Can you work these out from the model? Positions are in its coordinate system, mm. Face numbers are marked on the shaded views. Give positions to 0.01 mm unless a question says otherwise; leave off trailing zeros. Order: outer loops, then holes, each group sorted by start corner. A loop starts at its lowest first (then second) coordinate and runs counter-clockwise, first axis right, second up. Notation, with made-up numbers: (53.25, -6) -> (78.25, -6) arc R31 cw to (78.25, 32) -> close; hole circle Ø8 at (58.5, -19.5). An arc over 180 degrees is marked (long way). Answer as a JSON object with one key per item and string values.
Autodesk Inventor part; units mm, degrees
ref_plane "YZ Plane" through (0, 0, 0) normal (1, 0, 0) x (0, 1, 0)
ref_plane "XZ Plane" through (0, 0, 0) normal (0, 1, 0) x (-1, 0, 0)
ref_plane "XY Plane" through (0, 0, 0) normal (0, 0, 1) x (1, 0, 0)
sketch "스케치1" plane through (0, 0, 0) normal (1, 0, 0) x (0, 1, 0)
  line L0 (0, 0) -> (0, 20)
  line L1 (0, 20) -> (0, 50)
  line L2 (0, 0) -> (37.3205, 0)
  line L3 (0, 20) -> (17.3205, 20)
  line L4 (0, 50) -> (17.3205, 20)
  line L5 (0, 50) -> (34.641, 50) construction
  line L6 (17.3205, 20) -> (37.3205, 0)
  line L7 (17.3205, 20) -> (45.6048, 20) construction
  dimension "d0" = 20
  dimension "d1" = 30
  dimension "d2" = 60
  dimension "d3" = 45
extrude "돌출1" add sketch "스케치1" along normal blind 8
sketch "스케치2" plane through (8, 0, 0) normal (1, 0, 0) x (0, 0, -1)
  line L0 (-20, 17.3205) -> (-50, 0)
  line L1 (-50, 0) -> (0, 0)
  line L2 (0, 0) -> (0, 37.3205)
  line L3 (0, 37.3205) -> (-20, 17.3205)
  line L4 (-35.0718, 4) -> (-17.5439, 14.1197)
  line L5 (-17.5439, 14.1197) -> (-4, 27.6637)
  line L6 (-4, 27.6637) -> (-4, 4)
  line L7 (-4, 4) -> (-35.0718, 4)
  dimension "d6" = 4
extrude "돌출2" cut sketch "스케치2" against normal blind 8 contours L4 L5 L6 L7
sketch "스케치5" plane through (0, 0, 0) normal (0, -1, 0) x (1, 0, 0)
  arc A0 (157.7, 33) -> (156.7, 34) centre (156.7, 33) ccw
  line L0 (157.7, 33) -> (157.7, 24)
  arc A1 (156.7, 23) -> (157.7, 24) centre (156.7, 24) ccw
  line L1 (156.7, 23) -> (136.7, 23)
  arc A2 (135.7, 24) -> (136.7, 23) centre (136.7, 24) ccw
  line L2 (135.7, 24) -> (135.7, 33)
  arc A3 (136.7, 34) -> (135.7, 33) centre (136.7, 33) ccw
  line L3 (136.7, 34) -> (156.7, 34)
  arc A4 (-61.9, 33) -> (-62.9, 34) centre (-62.9, 33) ccw
  line L4 (-61.9, 33) -> (-61.9, 24)
  arc A5 (-62.9, 23) -> (-61.9, 24) centre (-62.9, 24) ccw
  line L5 (-62.9, 23) -> (-82.9, 23)
  arc A6 (-83.9, 24) -> (-82.9, 23) centre (-82.9, 24) ccw
  line L6 (-83.9, 24) -> (-83.9, 33)
  arc A7 (-82.9, 34) -> (-83.9, 33) centre (-82.9, 33) ccw
  line L7 (-82.9, 34) -> (-62.9, 34)
  arc A8 (-61.9, -244) -> (-62.9, -243) centre (-62.9, -244) ccw
  line L8 (-61.9, -244) -> (-61.9, -253)
  arc A9 (-62.9, -254) -> (-61.9, -253) centre (-62.9, -253) ccw
  line L9 (-62.9, -254) -> (-82.9, -254)
  arc A10 (-83.9, -253) -> (-82.9, -254) centre (-82.9, -253) ccw
  line L10 (-83.9, -253) -> (-83.9, -244)
  arc A11 (-82.9, -243) -> (-83.9, -244) centre (-82.9, -244) ccw
  line L11 (-82.9, -243) -> (-62.9, -243)
  arc A12 (136.7, -243) -> (135.7, -244) centre (136.7, -244) ccw
  line L12 (136.7, -243) -> (156.7, -243)
  arc A13 (157.7, -244) -> (156.7, -243) centre (156.7, -244) ccw
  line L13 (157.7, -244) -> (157.7, -253)
  arc A14 (156.7, -254) -> (157.7, -253) centre (156.7, -253) ccw
  line L14 (156.7, -254) -> (136.7, -254)
  arc A15 (135.7, -253) -> (136.7, -254) centre (136.7, -253) ccw
  line L15 (135.7, -253) -> (135.7, -244)
  line L16 (-98.1, 40) -> (171.9, 40)
  line L17 (-98.1, 0) -> (-98.1, 40)
  line L18 (-58.1, 0) -> (-98.1, 0)
  line L19 (-58.1, -220) -> (-58.1, 0)
  line L20 (-98.1, -220) -> (-58.1, -220)
  line L21 (-98.1, -260) -> (-98.1, -220)
  line L22 (171.9, -260) -> (-98.1, -260)
  line L23 (171.9, -220) -> (171.9, -260)
  line L24 (131.9, -220) -> (171.9, -220)
  line L25 (131.9, 0) -> (131.9, -220)
  line L26 (171.9, 0) -> (131.9, 0)
  line L27 (171.9, 40) -> (171.9, 0)
  circle A16 centre (4, 14.0286) radius 1.25
  circle A17 centre (4, 36.0286) radius 1.25
  point P0 (0, 0)
  dimension "d17" = 2.5
  dimension "d18" = 2.5
extrude "돌출5" cut sketch "스케치5" against normal blind 4.1 contours A16 | A17
sketch "스케치8" plane through (0, 17.3205, 20) normal (0, 0.7071, 0.7071) x (1, 0, 0)
  circle A0 centre (4, 8.6869) radius 1.5
  circle A1 centre (4, 18.6869) radius 1.5
  circle A2 centre (4, 18.6869) radius 1.25
  circle A3 centre (4, 8.6869) radius 1.25
  point P0 (0, 1.8947)
  dimension "d35" = 2.5
  dimension "d36" = 2.5
extrude "돌출7" cut sketch "스케치8" against normal blind 4.1 contours A2 | A3
sketch "스케치9" plane through (0, 0, 50) normal (0, 0.866, 0.5) x (1, 0, 0)
  circle A0 centre (4, 26) radius 1.5
  circle A1 centre (4, 16) radius 1.5
  circle A2 centre (4, 26) radius 1.25
  circle A3 centre (4, 16) radius 1.25
  point P0 (0, 43.3013)
  dimension "d39" = 2.5
  dimension "d40" = 2.5
extrude "돌출8" cut sketch "스케치9" against normal blind 4.1 contours A2 | A3
sketch "스케치10" plane through (8, 0, 0) normal (1, 0, 0) x (0, 0, -1)
  line L0 (-35.037, 4.1) -> (-35.037, 4.1)
  line L1 (-35.0184, 4.0308) -> (-35.037, 4.1)
  line L2 (-35.0184, 4.0308) -> (-35.0184, 4.0308)
  line L3 (-35.037, 4.1) -> (-35.0184, 4.0308)
  line L4 (-37.2261, 7.375) -> (-35.0611, 8.625)
  line L5 (-24.4008, 10.1609) -> (-26.5659, 8.9109)
  line L6 (-28.5659, 12.375) -> (-26.4008, 13.625)
  line L7 (-10.1451, 21.5185) -> (-11.9129, 19.7508)
  line L8 (-14.7413, 22.5792) -> (-12.9735, 24.347)
  line L9 (-7.6702, 29.6503) -> (-5.9025, 31.418)
  line L10 (-4, 27.5222) -> (-4, 27.6637)
  line L11 (-4, 27.5222) -> (-4, 27.5222)
  line L12 (-4, 27.6637) -> (-4, 27.5222)
  line L13 (-4, 27.6637) -> (-4, 27.6637)
  line L14 (-15.2786, 4) -> (-12.7786, 4)
  line L15 (-12.7786, 0) -> (-15.2786, 0)
  line L16 (-35.037, 4.1) -> (-35.0184, 4.0308)
  line L17 (-35.0718, 4) -> (-35.0184, 4.0308)
  line L18 (-35.0102, 4) -> (-35.0718, 4)
  line L19 (-35.0102, 4) -> (-34.9916, 3.9308)
  line L20 (-34.9916, 3.9308) -> (-34.8718, 4)
  line L21 (-34.8718, 4) -> (-34.8718, 4)
  line L22 (-34.8718, 4) -> (-34.9916, 3.9308)
  line L23 (-34.9916, 3.9308) -> (-35.0102, 4)
  line L24 (-35.0718, 4) -> (-35.0102, 4)
  line L25 (-35.0184, 4.0308) -> (-35.0718, 4)
  line L26 (-35.0184, 4.0308) -> (-35.037, 4.1)
  line L27 (-35.037, 4.1) -> (-35.037, 4.1)
  line L28 (-34.7786, 0) -> (-37.2786, 0)
  arc A0 (-36.7164, 7.6693) -> (-35.5708, 8.3307) centre (-36.5186, 8.6495) ccw
  arc A1 (-28.0562, 12.6693) -> (-26.9105, 13.3307) centre (-27.8583, 13.6495) ccw
  arc A2 (-14.3251, 22.9954) -> (-13.3897, 23.9308) centre (-14.3878, 23.9934) ccw
  arc A3 (-7.2541, 30.0664) -> (-6.3187, 31.0019) centre (-7.3167, 31.0645) ccw
  arc A4 (-13.196, 0) -> (-14.5189, 0) centre (-13.8574, -0.75) ccw
  arc A5 (-35.3671, 0) -> (-36.69, 0) centre (-36.0286, -0.75) ccw
  point P0 (0, 0)
  dimension "d43" = 2
  dimension "d44" = 2
  dimension "d45" = 2
  dimension "d46" = 2
  dimension "d47" = 2
  dimension "d48" = 2
  dimension "d49" = 0.75
  dimension "d50" = 0.75
  dimension "d51" = 0.75
  dimension "d52" = 0.75
  dimension "d53" = 0.75
  dimension "d54" = 0.75
extrude "돌출9" cut sketch "스케치10" against normal blind 8
properties part number "칼팁중간받침대" material "알루미늄 6061"
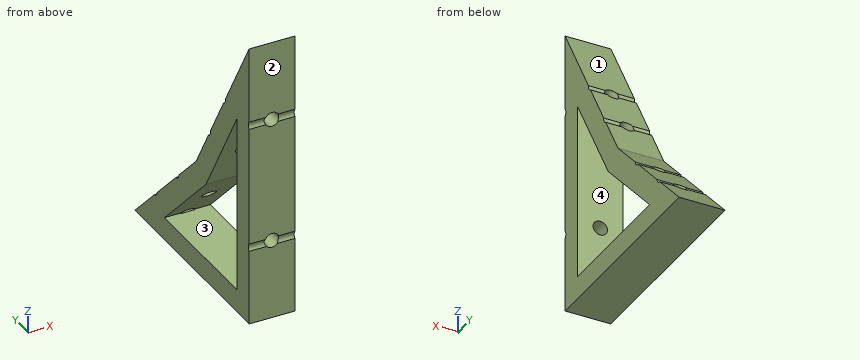
1. If we section it at A-A on x = 7: Please give me the cut outline in (y, z), then the cut area to 3 significant figures.
Worked answers:
{"outline": "(0, 0) -> (37.32, 0) -> (31, 6.32) arc R1 cw to (30.07, 7.25) -> (23.93, 13.39) arc R1 cw to (23, 14.33) -> (17.32, 20) -> (13.33, 26.91) arc R1 cw to (12.67, 28.06) -> (8.33, 35.57) arc R1 cw to (7.67, 36.72) -> (0, 50) -> (0, 36.69) arc R1 cw to (0, 35.37) -> (0, 14.52) arc R1 cw to (0, 13.2) -> close; hole (4, 4) -> (27.66, 4) -> (14.12, 17.54) -> (4, 35.07) -> close", "area": "487 mm²"}
2. If we section it at C-C on y = 6.5: Count the separate pieces of the cut face and the enclosed holes in it, then the cut area to 3 significant figures.
Worked answers:
{"separate pieces": "2", "enclosed holes": "1", "area": "90.3 mm²"}
3. If we mould it in two halves opening along Z, with no side actions, what happens to the marked faces 1, 2, 3 and 4? For each: +Z half, -Z half, draft (parallel to the pull), parting line (faces both ways), or undercut.
Worked answers:
{"face 1": "+Z half", "face 2": "draft", "face 3": "undercut", "face 4": "undercut"}
4. If we section it at B-B on z = 17: Please give me the cut outline in (x, y).
Worked answers:
{"outline": "(0, 0) -> (8, 0) -> (8, 4) -> (0, 4) -> close; (0, 14.66) -> (8, 14.66) -> (8, 20.32) -> (0, 20.32) -> close"}
5. Please list where these lines run through material, in increasing order: L1, parallel to Z at x = 4.75, y = 6.5; L2, parallel to Z at x = 4, y = 1.7; L3, parallel to X at y = 3.5, z = 35.
Worked answers:
{"L1": "0 to 4, 30.74 to 34.12, 36.43 to 38.74", "L2": "0 to 12.78, 15.28 to 34.78, 37.28 to 47.06", "L3": "0 to 3.29, 4.71 to 8"}
6. Will these pins go through, and if not, where does the flat tip stop? pin 1 Ø4 at (x, z) = (6, 14) entering from +Y; pin 2 Ø1.5 at (x, z) = (4, 36.03) entering from -Y; pin 3 Ø4 at (x, y) = (7, 23.5) entering from +Z.
Worked answers:
{"pin 1": "y = 25.32", "pin 2": "y = 4.1", "pin 3": "z = 15.82"}
